```python
from build123d import *

# Parameters (mm, degrees)
SKETCH_3_R          = 5
CUT_EXTRUDE_1_DEPTH = 228.266363547
CHAMFER_1_SIZE      = 0.5


with BuildPart() as part:
    # 草图1 → 旋转1 (revolve)
    with BuildSketch(Plane.XY, mode=Mode.PRIVATE) as revolve_1_sk:
        Polygon((0, 0), (0, 120), (6, 120), (6, 155), (22, 155), (22, 136), (66, 136), (66, 0), align=None)
    revolve(revolve_1_sk.sketch.rotate(Axis((0, 0, 0), (1, 0, 0)), 90), axis=Axis((0, 0, 0), (1, 0, 0)))

    # 草图2 → 切除-旋转1 (revolve, cut)
    with BuildSketch(Plane.XY, mode=Mode.PRIVATE) as cut_revolve_1_sk:
        Polygon((0, 0), (0, 95), (14, 95), (14, 90), (19, 90), (19, 112.5), (22, 112.5), (22, 120), (59, 120), (59, 121.5), (61.5, 121.5), (61.5, 120), (66, 120), (66, 0), align=None)
    revolve(cut_revolve_1_sk.sketch.rotate(Axis((0, 0, 0), (1, 0, 0)), 90), axis=Axis((0, 0, 0), (1, 0, 0)), mode=Mode.SUBTRACT)

    # 草图3 → 切除-拉伸1 (cut, through all)
    with BuildSketch(Plane.ZY.offset(-6)):
        with Locations((0, 145)):
            Circle(SKETCH_3_R)
        with Locations((72.5, 125.573683549)):
            Circle(SKETCH_3_R)
        with Locations((125.573683549, 72.5)):
            Circle(SKETCH_3_R)
        with Locations((145, 0)):
            Circle(SKETCH_3_R)
        with Locations((125.573683549, -72.5)):
            Circle(SKETCH_3_R)
        with Locations((72.5, -125.573683549)):
            Circle(SKETCH_3_R)
        with Locations((0, -145)):
            Circle(SKETCH_3_R)
        with Locations((-72.5, -125.573683549)):
            Circle(SKETCH_3_R)
        with Locations((-125.573683549, -72.5)):
            Circle(SKETCH_3_R)
        with Locations((-145, 0)):
            Circle(SKETCH_3_R)
        with Locations((-125.573683549, 72.5)):
            Circle(SKETCH_3_R)
        with Locations((-72.5, 125.573683549)):
            Circle(SKETCH_3_R)
    extrude(amount=-CUT_EXTRUDE_1_DEPTH, mode=Mode.SUBTRACT)

    # 倒角1
    chamfer_1_edges = [part.edges().sort_by_distance(p)[0] for p in [
        (0, 0, -95),
        (66, 0, -136),
        (22, 0, -155),
    ]]
    chamfer(chamfer_1_edges, length=CHAMFER_1_SIZE)


solid = part.part
```
Input: part model. Units: mm. Frame: model coordinates. A direction names the side the tool comes from. Give positions to 0.01 mm unless a question says otherwise; leave off trailing zeros. Write each loop counter-clockwise with the first axis right and the second up, starting at its lowest first coordinate (ties: lowest second). Pieces come first, ordered by that corner, then holes. Notation, with made-up numbers: (71.5, 21) - (130.5, 21) arc R10 ccw to (130.5, 39) - close; hole circle Ø4 at (-19.5, -32.75). An arc over 180 degrees is marked (long way). Write item = value, one per line. Start each with the question number.
1) Reachability of faces 1 (the face through (13.89, -130.01, -70.19)), 2 (the face through (6, -116, 35)), 3 (the face through (66, 120, -11)), 4 (the face through (60.268, 107.791, 56.065)), 5 (the face through (22, -107.2, -35)) from +Z, -Z, +X, -X, +Y, -Y: full face, straight path, thin tool, end or side. Return the list, or none.
2) Material intervals for L1, parallel to Z at x = 50, y = -4; L2, parallel to Y at x = 60.3, z = 0; L3, parallel to Y at x = 20.7, z = 0, sorted ascending. Write a range as [from, to].
3) Pin query (flat end, axial travel): pin 1 (8 mm diameter, centred on x = 48, z = -10.5, fed in from +Y); pin 2 (5 mm diameter, centred on x = 36.5, z = -65, fed in from -Y); pin 3 (9 mm diameter, centred on y = 72.5, z = 125.57, fed in from +X); pin 4 (2 mm diameter, centred on x = 11.5, y = 25.5, fed in from +Z). Return the tip coordinate at first contact, or that it passes through.
4) Draft query along Y for faces 6 (the face through (22, 137, -1)), 7 (the face through (13.9, -74.4, 130.2)), 8 (the face through (44.055, -134.843, -17.704)). Return one class per face: pulls with the +Y half, pulls with the -Y half, needs draft (parallel to the pull), parting line crosses it, or undercut.
5) Cut plane A-A (z = 0). Give the number of separate pieces and of enclosed holes in the cut face, and give its area (3 significant figures).
6) Cut plane C-C (x = 46). Return loops of the section in (y, z), and give its area (3 significant figures).
Answers follow:
q1.face_1 = +X, -X
q1.face_2 = -X
q1.face_3 = +Z, -Z, +X, +Y, -Y
q1.face_4 = none
q1.face_5 = +X
q2.L1 = [-135.94, -119.93], [119.93, 135.94]
q2.L2 = [-136, -121.5], [121.5, 136]
q2.L3 = [-155, -150], [-140, -112.5], [112.5, 140], [150, 155]
q3.pin_1 = 135.84
q3.pin_2 = -120.79
q3.pin_3 = through
q3.pin_4 = 153.05
q4.face_6 = needs draft
q4.face_7 = undercut
q4.face_8 = parting line crosses it
q5.separate_pieces = 4
q5.enclosed_holes = 0
q5.area = 3,240 mm^2
q6.outline = circle Ø272 at (0, 0); hole circle Ø240 at (0, 0)
q6.area = 12,900 mm^2
